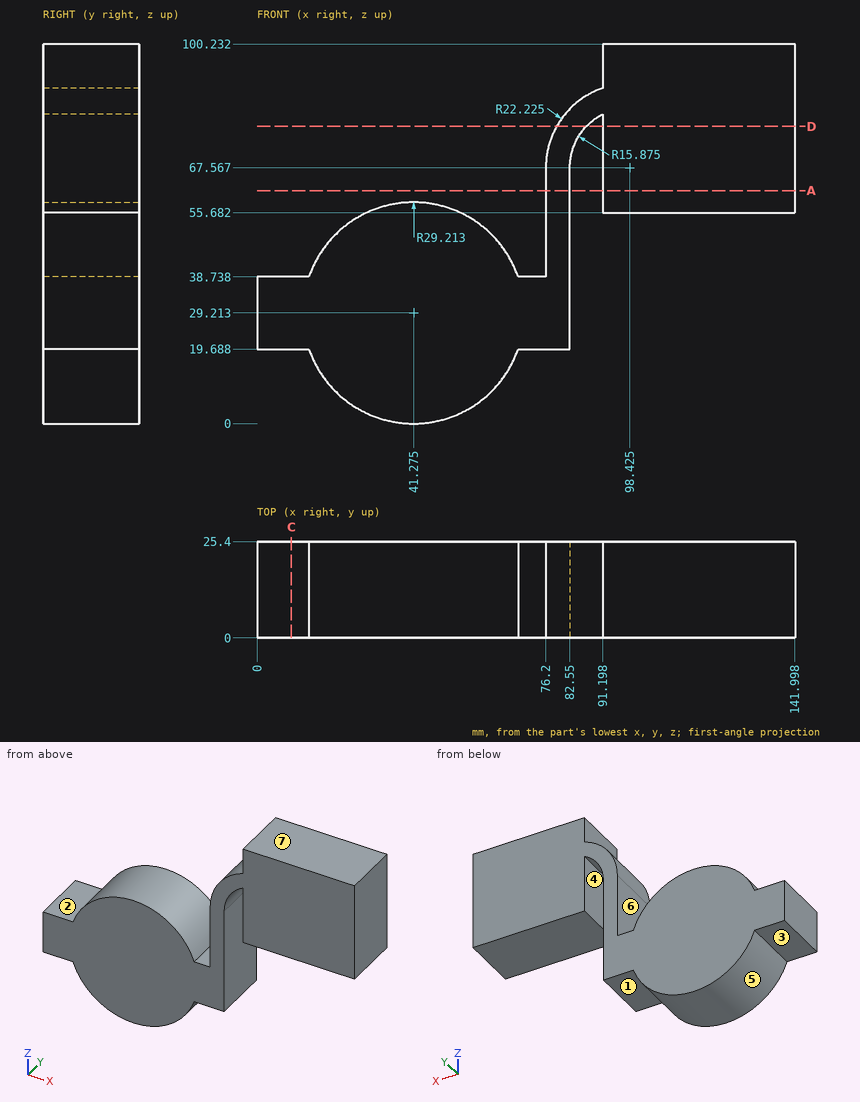
Could you check a few things on this drawing? It's one solid part, dimensions in mm from its lowest x, y, z. A direction names the side the tool comes from. Round coordinates to 2 decimals unless told otherwise and drop trailing zeros. Write each loop counter-clockwise with the first axis right and the second up, starting at its lowest first coordinate (ties: lowest second). Pieces come first, ordered by that corner, then holes.
Q1. If we section it at D-D on z = 78.5: Write out the boundary of the cut face in (x, y) (1 decimal).
Q2. Will these pins go through, and if not, where does the flat tip stop? P1, Ø5, axis at y = 2.5, z = 70, coming from the -X side; P2, Ø7.5, axis at y = 7.5, z = 38, coming from the +X side; P3, Ø4, axis at x = 62.5, y = 6.5, coming from the -Z side.
Q3. Which directions (+Z, -Z, +X, -X, +Y, -Y) give clear straight access to the entire face, cutting with the end or side of a thin tool? Please do the marked faces 1, 2, 3 and 4.
Q4. If we section it at A-A on z = 61.5: Write out the boundary of the cut face in (x, y).
Q5. If we mould it in two halves opening along X, with no side actions, what happens to the marked faces 5, 6 and 7? For each: +X half, -X half, draft (parallel to the pull), parting line (faces both ways), or undercut.
Q6. Please list where these lines run through material, in increasing order: probe 1 along X at (y, z) = (19.75, 59.5); probe 2 along X at (y, z) = (8, 94); probe 3 along Z at (x, y) = (127.5, 12.5).
Q7. If we section it at C-C on x = 9: Write out the boundary of the cut face in (y, z), plus the area to 3 significant figures.
Answer below:
1. outline: (79.1, 0) - (86.9, 0) - (86.9, 25.4) - (79.1, 25.4) - close; (91.2, 0) - (142, 0) - (142, 25.4) - (91.2, 25.4) - close
2. P1: stops at x = 76.2
2. P2: stops at x = 82.55
2. P3: stops at z = 7.22
3. face 1: -Z, +X, +Y, -Y
3. face 2: +Z, -X, +Y, -Y
3. face 3: -Z, -X, +Y, -Y
3. face 4: -Z, +Y, -Y
4. outline: (76.2, 0) - (82.55, 0) - (82.55, 25.4) - (76.2, 25.4) - close; (91.2, 0) - (142, 0) - (142, 25.4) - (91.2, 25.4) - close
5. face 5: parting line
5. face 6: undercut
5. face 7: draft
6. probe 1: x = 76.2 to 82.55, 91.2 to 142
6. probe 2: x = 91.2 to 142
6. probe 3: z = 55.68 to 100.23
7. outline: (0, 19.69) - (25.4, 19.69) - (25.4, 38.74) - (0, 38.74) - close
7. area: 484 mm2
